from build123d import *

# Parameters (mm, degrees)
SKETCH1_W           = 74.93
SKETCH1_H           = 40.132
SKETCH1_W_2         = 69.85
SKETCH1_H_2         = 35.052
BOSS_EXTRUDE1_DEPTH = 5.08
SKETCH2_W           = 74.93
SKETCH2_H           = 77.724
BOSS_EXTRUDE2_DEPTH = 2.54
SKETCH3_W           = 8.89
SKETCH3_H           = 77.724
BOSS_EXTRUDE3_DEPTH = 6.35
SKETCH5_W           = 12.7
SKETCH5_H           = 13.97
BOSS_EXTRUDE5_DEPTH = 12.7
SKETCH6_W           = 12.7
SKETCH6_H           = 13.97
BOSS_EXTRUDE6_DEPTH = 12.7
CHAMFER2_SIZE       = 12.7
CHAMFER2_SIZE_2     = 14.104778938
SKETCH7_R           = 2.54
CUT_EXTRUDE1_DEPTH  = 78.614252678
CUT_EXTRUDE2_START  = -2.54
SKETCH8_R           = 5.08
CUT_EXTRUDE2_DEPTH  = 76.074252678
FILLET1_R           = 2.38


with BuildPart() as part:
    # Sketch1 → Boss-Extrude1 (new body)
    # profile 1 of 2: a face of its own
    with BuildSketch(Plane(origin=(0, 0, 0), x_dir=(1, 0, 0), z_dir=(0, 1, 0))):
        Polygon((-37.465, 57.658), (-37.465, 20.066), (-34.925, 20.066), (-34.925, 55.118), (34.925, 55.118), (34.925, 20.066), (37.465, 20.066), (37.465, 57.658), align=None)
    # profile 2 of 2: a face of its own
    with BuildSketch(Plane(origin=(0, 0, 0), x_dir=(1, 0, 0), z_dir=(0, 1, 0))):
        Rectangle(SKETCH1_W, SKETCH1_H)
        Rectangle(SKETCH1_W_2, SKETCH1_H_2, mode=Mode.SUBTRACT)
    extrude(amount=BOSS_EXTRUDE1_DEPTH)

    # Sketch2 → Boss-Extrude2 (add)
    with BuildSketch(Plane.XZ):
        with Locations((0, -18.796)):
            Rectangle(SKETCH2_W, SKETCH2_H)
    extrude(amount=BOSS_EXTRUDE2_DEPTH)

    # Sketch3 → Boss-Extrude3 (add)
    with BuildSketch(Plane(origin=(0, -2.54, 0), x_dir=(-1, 0, 0), z_dir=(0, -1, 0))):
        with Locations((-33.02, 18.796)):
            Rectangle(SKETCH3_W, SKETCH3_H)
        with Locations((33.02, 18.796)):
            Rectangle(SKETCH3_W, SKETCH3_H)
    extrude(amount=BOSS_EXTRUDE3_DEPTH)

    # Sketch5 → Boss-Extrude5 (add)
    with BuildSketch(Plane(origin=(37.465, 0, 0), x_dir=(0, 0, -1), z_dir=(1, 0, 0))):
        with Locations((51.308, -1.905)):
            Rectangle(SKETCH5_W, SKETCH5_H)
        with Locations((-13.716, -1.905)):
            Rectangle(SKETCH5_W, SKETCH5_H)
    extrude(amount=BOSS_EXTRUDE5_DEPTH)

    # Sketch6 → Boss-Extrude6 (add)
    with BuildSketch(Plane.ZY.offset(37.465)):
        with Locations((-51.308, -1.905)):
            Rectangle(SKETCH6_W, SKETCH6_H)
        with Locations((13.716, -1.905)):
            Rectangle(SKETCH6_W, SKETCH6_H)
    extrude(amount=BOSS_EXTRUDE6_DEPTH)

    # Chamfer2
    # the kernel refuses this chamfer: 14.104778938, 12.7 mm, written as the material it takes off along each edge
    with BuildSketch(Plane(origin=(50.165, 5.08, -28.95640044), x_dir=(-0.9994864482690293, 0.03204434000819555, 0), z_dir=(0, 0, 1))) as chamfer2_piece_1:
        Polygon((CHAMFER2_SIZE * 0.999486448269, CHAMFER2_SIZE * 0.0320443400082), (-CHAMFER2_SIZE_2 * 0.0320443400089, CHAMFER2_SIZE_2 * 0.999486448292), (0, 0), align=None)
    extrude(amount=85.34480088, mode=Mode.SUBTRACT)
    with BuildSketch(Plane(origin=(50.165, 5.08, -8.63559956), x_dir=(-0.9994864482690293, 0.03204434000819555, 0), z_dir=(0, 0, -1)), Plane(origin=(-50.165, 5.08, -28.95640044), x_dir=(0.9994864482690293, 0.03204434000819555, 0), z_dir=(0, 0, 1)), Plane(origin=(-50.165, 5.08, -93.98040044), x_dir=(0.9994864482690293, 0.03204434000819555, 0), z_dir=(0, 0, 1))) as chamfer2_piece_2:
        Polygon((CHAMFER2_SIZE * 0.999486448269, -CHAMFER2_SIZE * 0.0320443400082), (-CHAMFER2_SIZE_2 * 0.0320443400089, -CHAMFER2_SIZE_2 * 0.999486448292), (0, 0), align=None)
    extrude(amount=85.34480088, mode=Mode.SUBTRACT)

    # Sketch7 → Cut-Extrude1 (cut, through all)
    with BuildSketch(Plane(origin=(0, -8.89, 0), x_dir=(-1, 0, 0), z_dir=(0, -1, 0))):
        with Locations(Location((-43.693644499, 51.308, 0), (0, 0, 90))):
            Circle(SKETCH7_R)
        with Locations(Location((-43.693644499, -13.716, 0), (0, 0, 90))):
            Circle(SKETCH7_R)
        with Locations(Location((43.693644499, -13.716, 0), (0, 0, 90))):
            Circle(SKETCH7_R)
        with Locations(Location((43.693644499, 51.308, 0), (0, 0, 90))):
            Circle(SKETCH7_R)
    extrude(amount=-CUT_EXTRUDE1_DEPTH, mode=Mode.SUBTRACT)

    # Sketch8 → Cut-Extrude2 (cut, through all)
    with BuildSketch(Plane(origin=(0, -8.89, 0), x_dir=(-1, 0, 0), z_dir=(0, -1, 0)).offset(CUT_EXTRUDE2_START)):
        with Locations((-43.693644499, 51.308)):
            Circle(SKETCH8_R)
        with Locations((-43.693644499, -13.716)):
            Circle(SKETCH8_R)
        with Locations((43.693644499, -13.716)):
            Circle(SKETCH8_R)
        with Locations((43.693644499, 51.308)):
            Circle(SKETCH8_R)
    extrude(amount=-CUT_EXTRUDE2_DEPTH, mode=Mode.SUBTRACT)

    # Fillet1
    fillet1_edges = [part.edges().sort_by_distance(p)[0] for p in [
        (28.575, -2.54, -18.796),
        (-28.575, -2.54, -18.796),
    ]]
    fillet(fillet1_edges, radius=FILLET1_R)


solid = part.part
Geometry check sheet. Reference: the model listing, model coordinates, mm. A direction names the side the tool comes from. Give positions to 0.01 mm unless a question says otherwise; leave off trailing zeros. Loops run counter-clockwise (first coordinate to the right, second up) from the corner with the lowest first, then second, coordinate; pieces in that order, holes last.
(1) Section check A-A on z = -32. Record the cut outline in (x, y) (3 decimals).
From the geometry:
outline: (-37.465, -8.89) - (-28.575, -8.89) - (-28.575, -4.92) arc R2.38 cw to (-26.195, -2.54) - (26.195, -2.54) arc R2.38 cw to (28.575, -4.92) - (28.575, -8.89) - (37.465, -8.89) - (37.465, 5.08) - (34.925, 5.08) - (34.925, 0) - (-34.925, 0) - (-34.925, 5.08) - (-37.465, 5.08) - close
(2) Section check D-D on x = -32.5. Record the cut outline in (y, z), then the cut area to 3 significant figures.
From the geometry:
outline: (-8.89, -57.66) - (5.08, -57.66) - (5.08, -55.12) - (0, -55.12) - (0, -20.07) - (5.08, -20.07) - (5.08, -17.53) - (0, -17.53) - (0, 17.53) - (5.08, 17.53) - (5.08, 20.07) - (-8.89, 20.07) - close
area: 730 mm2
(3) Set-up check for faces 4 (the flat face through (-37.465, -2, -19)), 5 (the cylindrical face through (42.15, -7.64, -49.29)), 6 (the flat face through (-28.575, -7, -18)), 7 (the flat face through (0, 3, -55.118)), 8 (the flat face through (42, -4, -44.958)): record each of +Z, -Z, +X, -X, +Y, -Y from which the full face is reachable in a straight line by a thin tool's end or side.
From the geometry:
face 4: -X, +Y, -Y
face 5: +Y, -Y
face 6: +Z, -Z, -Y
face 7: +Y
face 8: +X, +Y, -Y
(4) Release check for a two-part mould opening along X. For faces 1 (the flat face through (37.465, -2, -18)), 2 (the flat face through (0, 3, -20.066)), 3 (the flat face through (42, -4, 7.366)) record: released by +X, released by -X, zero draft, split by the parting line, or undercut.
From the geometry:
face 1: released by +X
face 2: undercut
face 3: zero draft
(5) Depth check by flat-ended pin: pin 1 Ø2 at (x, z) = (16.5, -32) entering from -Y; pin 2 Ø2.5 at (y, z) = (2.5, 8.5) entering from -X; pin 3 Ø2.5 at (y, z) = (1.5, -31.5) entering from +X (3 decimals); pin 4 Ø3 at (x, z) = (43.69, 13.72) entering from -Y. Enter the tip coordinate at first touch or a pass-through.
From the geometry:
pin 1: stops at y = -2.54
pin 2: stops at x = -40.91
pin 3: stops at x = 37.465
pin 4: passes through
(6) Section check B-B on x = -16.5. Record the cut outline in (y, z).
From the geometry:
outline: (-2.54, -57.66) - (5.08, -57.66) - (5.08, -55.12) - (0, -55.12) - (0, -20.07) - (5.08, -20.07) - (5.08, -17.53) - (0, -17.53) - (0, 17.53) - (5.08, 17.53) - (5.08, 20.07) - (-2.54, 20.07) - close
(7) Thickness scan on L1, parallel to Z at x = 16, y = 3.5; L2, parallel to X at y = -5, z = -13 (3 decimals); L3, parallel to Z at x = 41.5, y = -2.5. Record the ranges inside material, lowest first.
From the geometry:
L1: z = -57.66 to -55.12, -20.07 to -17.53, 17.53 to 20.07
L2: x = -37.465 to -28.575, 28.575 to 37.465
L3: z = -57.66 to -55.89, -46.73 to -44.96, 7.37 to 9.13, 18.3 to 20.07
(8) Section check C-C on y = 1.75. Record the cut outline in (x, z) (3 decimals).
From the geometry:
outline: (-40.463, -57.658) - (40.463, -57.658) - (40.463, -55.229) arc R5.08 cw to (40.463, -47.387) - (40.463, -44.958) - (37.465, -44.958) - (37.465, 7.366) - (40.463, 7.366) - (40.463, 9.795) arc R5.08 cw to (40.463, 17.637) - (40.463, 20.066) - (-40.463, 20.066) - (-40.463, 17.637) arc R5.08 cw to (-40.463, 9.795) - (-40.463, 7.366) - (-37.465, 7.366) - (-37.465, -44.958) - (-40.463, -44.958) - (-40.463, -47.387) arc R5.08 cw to (-40.463, -55.229) - close; hole (-34.925, -55.118) - (34.925, -55.118) - (34.925, -20.066) - (-34.925, -20.066) - close; hole (-34.925, -17.526) - (34.925, -17.526) - (34.925, 17.526) - (-34.925, 17.526) - close
